The drawing under review shows one solid part. Ordinate dimensions are in mm from its lowest x, y, z. A direction names the side the tool comes from. Give positions to 0.01 mm unless a question says otherwise; leave off trailing zeros. Order: outer loops, then holes, each group sorted by start corner. A loop starts at its lowest first (then second) coordinate and runs counter-clockwise, first axis right, second up. Notation, with made-up numbers: (37.5, 61.5) -> (56.5, 61.5) arc R11 ccw to (56.5, 79.5) -> close; hole circle Ø11 at (48, -35.75). An arc over 180 degrees is marked (long way). Return JSON: item names as keys, results as strings. Group by question number.
1) For the marked faces 1, 2, 3 and 4, list the 3-axis set-ups (+Z, -Z, +X, -X, +Y, -Y) from which the entire face can be reached by the end or side of a thin tool; tool diameter is ignored.
2) To check wall thickness, follow line 1 along X through (y, z) = (26, 25); line 2 along Z through (x, y) = (30, 11). State the ranges of each line that lie inside material, in increasing order.
3) Insertion check: P1, Ø11, axis at x = 93.5, z = 31, coming from the -Y side; P2, Ø14, axis at y = 72.5, z = 20.5, coming from the -X side; P3, Ø17, axis at x = 9, y = 29, coming from the +Z side; P4, Ø16, axis at x = 32.5, z = 19, coming from the +Y side. Each pin has a flat end and moves straight along its axis. Give the tip position at first contact, or say it passes through.
4) Add section C-C (x = 43). Give the boundary of the cut face in (y, z), then the cut area to 3 significant figures.
5) The part is to be moulded in two halves that separate along X. For the marked faces 5, 6 and 7, say which applies: released by +X, released by -X, zero draft, split by the parting line, or undercut.
6) Add section A-A (y = 86.25). Give the boundary of the cut face in (x, z).
7) Add section D-D (x = 100). Give the boundary of the cut face in (y, z).
8) Add section B-B (y = 25.5). Give the boundary of the cut face in (x, z).
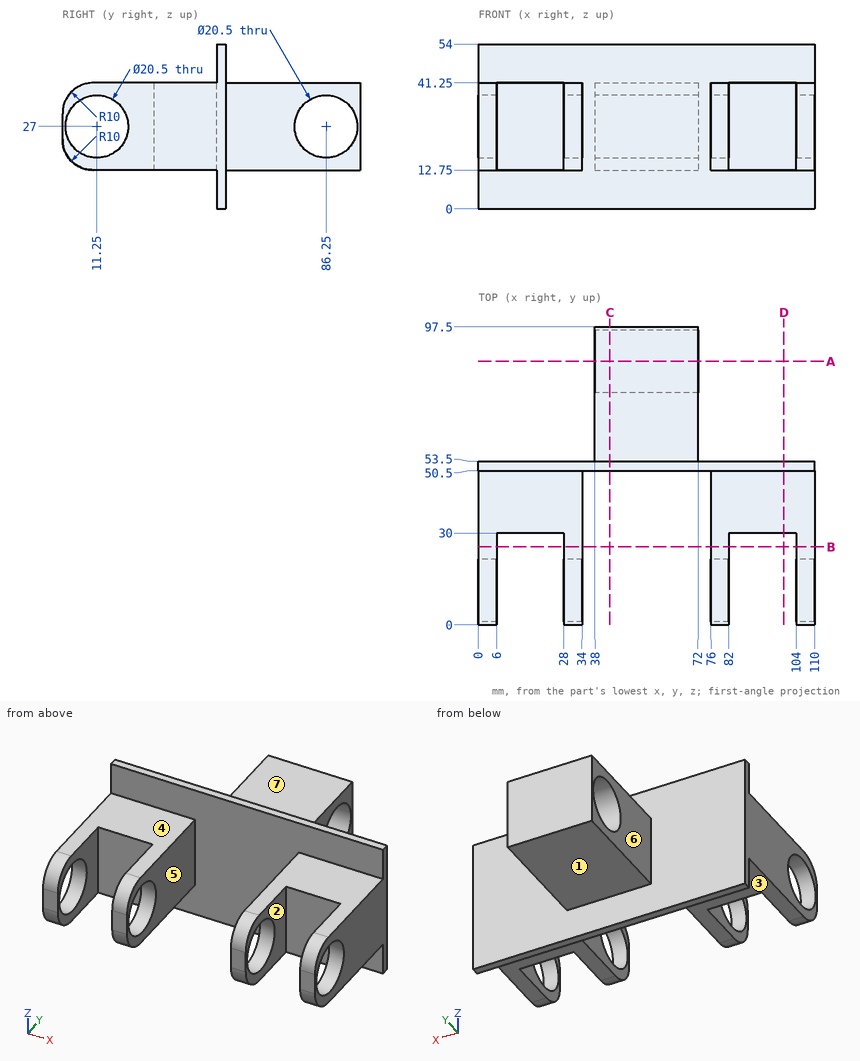
Evaluation:
{
 "1": {"face 1": "-Z, +X, -X, +Y", "face 2": "+Z, -Z, -Y", "face 3": "-Z, +X, -X, -Y", "face 4": "+Z, +X, -X, -Y"},
 "2": {"line 1": "0 to 6, 28 to 34, 76 to 82, 104 to 110", "line 2": "12.75 to 16.75, 37.25 to 41.25"},
 "3": {"P1": "y = 30", "P2": "x = 38", "P3": "z = 41.25", "P4": "y = 97.5"},
 "4": {"outline": "(50.5, 0) -> (53.5, 0) -> (53.5, 12.75) -> (97.5, 12.75) -> (97.5, 41.25) -> (53.5, 41.25) -> (53.5, 54) -> (50.5, 54) -> close; hole circle Ø20.5 at (86.25, 27)", "area": "1,090 mm^2"},
 "5": {"face 5": "undercut", "face 6": "released by -X", "face 7": "zero draft"},
 "6": {"outline": "(38, 12.75) -> (72, 12.75) -> (72, 16.75) -> (38, 16.75) -> close; (38, 37.25) -> (72, 37.25) -> (72, 41.25) -> (38, 41.25) -> close"},
 "7": {"outline": "(30, 12.75) -> (50.5, 12.75) -> (50.5, 0) -> (53.5, 0) -> (53.5, 54) -> (50.5, 54) -> (50.5, 41.25) -> (30, 41.25) -> close"},
 "8": {"outline": "(0, 12.75) -> (6, 12.75) -> (6, 41.25) -> (0, 41.25) -> close; (28, 12.75) -> (34, 12.75) -> (34, 41.25) -> (28, 41.25) -> close; (76, 12.75) -> (82, 12.75) -> (82, 41.25) -> (76, 41.25) -> close; (104, 12.75) -> (110, 12.75) -> (110, 41.25) -> (104, 41.25) -> close"}
}
